Autodesk Inventor part; units mm, degrees
ref_plane "YZ Plane" through (0, 0, 0) normal (1, 0, 0) x (0, 1, 0)
ref_plane "XZ Plane" through (0, 0, 0) normal (0, 1, 0) x (-1, 0, 0)
ref_plane "XY Plane" through (0, 0, 0) normal (0, 0, 1) x (1, 0, 0)
sketch "Sketch1" plane through (0, 0, 0) normal (0, 1, 0) x (-1, 0, 0)
  line L0 (-12.7, -12.7) -> (12.7, -12.7)
  line L1 (12.7, -12.7) -> (12.7, 12.7)
  line L2 (12.7, 12.7) -> (-12.7, 12.7)
  line L3 (-12.7, 12.7) -> (-12.7, -12.7)
  line L4 (-12.7, -12.7) -> (12.7, 12.7) construction
  line L5 (12.7, -12.7) -> (-12.7, 12.7) construction
  line L6 (9.525, 9.525) -> (9.525, -9.525)
  line L7 (9.525, -9.525) -> (-9.525, -9.525)
  line L8 (-9.525, -9.525) -> (-9.525, 9.525)
  line L9 (-9.525, 9.525) -> (9.525, 9.525)
  point P0 (0, 0)
  dimension "d0" = 25.4
  dimension "d1" = 25.4
  dimension "d2" = 3.175
extrude "Extrusion1" add sketch "Sketch1" along normal blind 420.5313
sketch "Sketch2" plane through (12.7, 0, -12.7) normal (0, 0, -1) x (-1, 0, 0)
  line L0 (0, 0) -> (25.4, 25.4)
  line L1 (25.4, 0) -> (25.4, 420.5313)
  line L2 (0, 0) -> (25.4, 0)
  line L3 (25.4, 0) -> (25.4, 420.5313)
  line L4 (0, 420.5313) -> (25.4, 420.5313)
  line L5 (0, 0) -> (0, 420.5313)
  line L6 (0, 420.5313) -> (25.4, 395.1313)
  point P0 (12.7, 0)
  dimension "d5" = 25.4
  dimension "d6" = 25.4
extrude "Extrusion2" cut sketch "Sketch2" against normal blind 451.1802 contours L0 L1 L2 | L4 L1 L6
sketch "Sketch3" plane through (12.7, 0, 12.7) normal (-0.7071, -0.7071, 0) x (-0.7071, 0.7071, 0)
  line L0 (35.921, 0) -> (0, 0)
  line L1 (35.921, 25.4) -> (35.921, 0)
  line L2 (0, 25.4) -> (35.921, 25.4)
  line L3 (0, 0) -> (0, 25.4)
  line L4 (4.4901, 3.175) -> (31.4309, 3.175)
  line L5 (4.4901, 22.225) -> (4.4901, 3.175)
  line L6 (31.4309, 22.225) -> (4.4901, 22.225)
  line L7 (31.4309, 3.175) -> (31.4309, 22.225)
  line L8 (35.921, 0) -> (297.3605, 0)
  line L9 (35.921, 0) -> (0, 25.4)
  line L10 (35.921, 25.4) -> (0, 0)
  circle A0 centre (17.9605, 12.7) radius 2.0193
  point P0 (8.9803, 12.7)
  dimension "d9" = 4.0386
extrude "Extrusion3" cut sketch "Sketch3" against normal through all contours A0 L10 L9 | L9 L10 A0 | A0 L9 L10 | L10 L9 A0
sketch "Sketch4" plane through (12.7, 420.5313, -12.7) normal (-0.7071, 0.7071, 0) x (-0.7071, -0.7071, 0)
  line L0 (0, 25.4) -> (35.921, 25.4) construction
  line L1 (0, 25.4) -> (0, 0) construction
  line L2 (35.921, 0) -> (0, 0) construction
  line L3 (35.921, 25.4) -> (35.921, 0) construction
  line L4 (31.4309, 22.225) -> (4.4901, 22.225) construction
  line L5 (31.4309, 3.175) -> (31.4309, 22.225) construction
  line L6 (4.4901, 3.175) -> (31.4309, 3.175) construction
  line L7 (4.4901, 22.225) -> (4.4901, 3.175) construction
  line L8 (0, 0) -> (35.921, 25.4) construction
  line L9 (35.921, 0) -> (0, 25.4) construction
  circle A0 centre (17.9605, 12.7) radius 2.0193
  point P0 (306.3408, 12.7)
  dimension "d12" = 4.0386
extrude "Extrusion4" cut sketch "Sketch4" against normal through all
thread "Thread1"
thread "Thread2"
properties part number "STRU_010_BilletCrossbar_17.7in_Angled" material "Aluminum 6061"
Model file for the job. Use its own axes, mm. A direction names the side the tool comes from. Give positions to 0.01 mm unless a question says otherwise; leave off trailing zeros. Order: outer loops, then holes, each group sorted by start corner. A loop starts at its lowest first (then second) coordinate and runs counter-clockwise, first axis right, second up.
1) 3-axis set-ups, long thin cutter, end or side, ignore diameter. For faces 4 (the flat face through (-9.525, 208, 0)), 5 (the flat face through (0.2, 12.5, 11.1)): which of +Z, -Z, +X, -X, +Y, -Y reach the whole face in a straight line?
2) Mould opens along Z. For faces 1 (the flat face through (0, 207, -12.7)), 2 (the flat face through (0.18, 408.01, 11.11)), 3 (the flat face through (0, 207, 9.525)) say: +Z half, -Z half, draft (parallel to the pull), parting line (faces both ways), or undercut.
3) Wall check: probe 1 along Z at (x, y) = (5.5, 134.5) (3 decimals); probe 2 along Y at (x, z) = (-3.25, -11.5). Give the ranges that are in metal, low to high.
4) Saw through at B-B, the plane y = 75.5. Write the cut outline in (x, z) (3 decimals).
5) Saw through at A-A, the plane z = -5.5. Write the cut outline in (x, y) (3 decimals).
6) Saw through at C-C, the plane x = -1. Write the cut outline in (y, z) (3 decimals), then the cut area to 3 significant figures.
Computed:
1. face 4: +Y, -Y
1. face 5: +Z, -Z, -X, -Y
2. face 1: -Z half
2. face 2: draft
2. face 3: undercut
3. probe 1: z = -12.7 to -9.525, 9.525 to 12.7
3. probe 2: y = 15.95 to 404.58
4. outline: (-12.7, -12.7) - (12.7, -12.7) - (12.7, 12.7) - (-12.7, 12.7) - close; hole (-9.525, -9.525) - (9.525, -9.525) - (9.525, 9.525) - (-9.525, 9.525) - close
5. outline: (-12.7, 25.4) - (-9.525, 22.225) - (-9.525, 398.306) - (-12.7, 395.131) - close; (9.525, 3.175) - (12.7, 0) - (12.7, 420.531) - (9.525, 417.356) - close
6. outline: (13.7, -12.7) - (406.831, -12.7) - (406.831, -9.525) - (13.7, -9.525) - close; (13.7, 9.525) - (406.831, 9.525) - (406.831, 12.7) - (13.7, 12.7) - close
6. area: 2,500 mm2
